Answer from the drawing. Dimensions are ordinates in mm from the lowest x, y and z of the part. A direction names the side the tool comes from. Coordinates: 2 decimals unless noted, no trailing zeros. Loops run counter-clockwise (first coordinate to the right, second up) from the corner with the lowest first, then second, coordinate; pieces in that order, holes last. Notation, with made-up numbers: (83, 68.25) -> (99, 68.25) arc R21 ccw to (99, 72.25) -> close; hole circle Ø2 at (-35, 59). An arc over 180 degrees is marked (long way). Use a Markdown table: item, result.
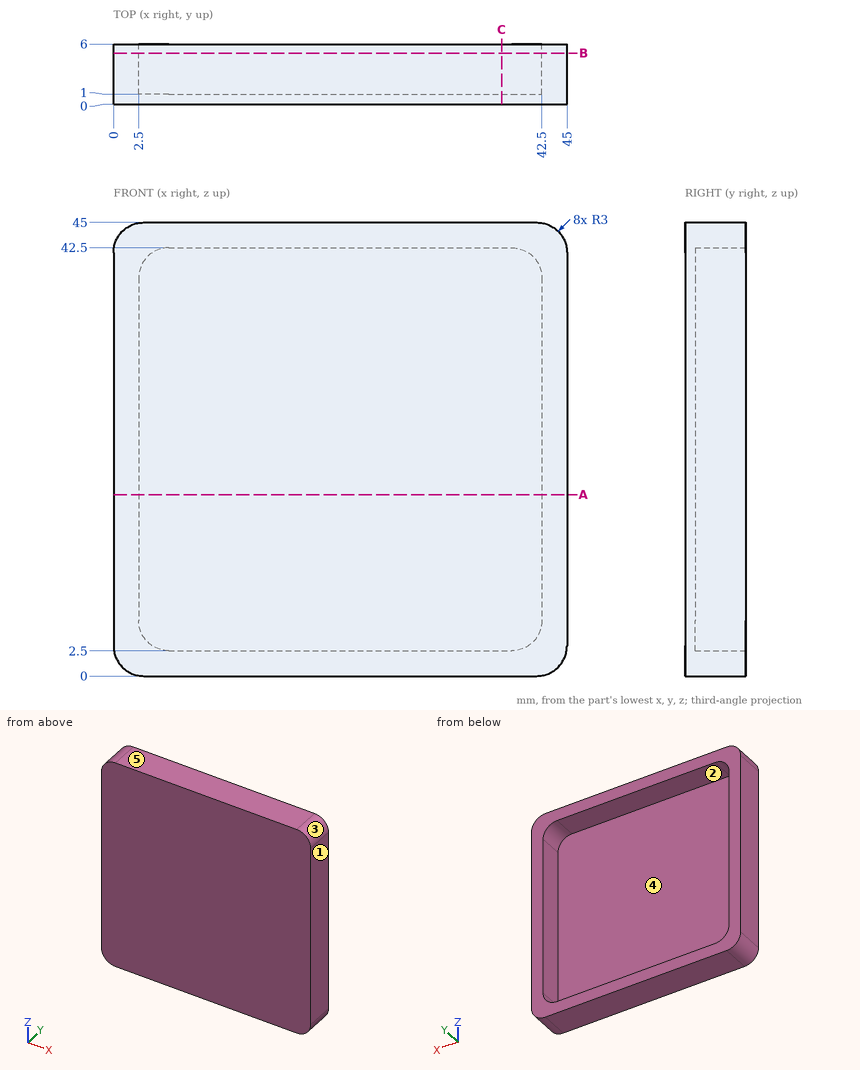
Q1. Section B-B on y = 5.1 is taken. Determine the outline of the cut face in (x, z), and give its area (3 significant figures).
Solved:
| item | result |
|---|---|
| outline | (0, 3) arc R3 ccw to (3, 0) -> (42, 0) arc R3 ccw to (45, 3) -> (45, 42) arc R3 ccw to (42, 45) -> (3, 45) arc R3 ccw to (0, 42) -> close; hole (2.5, 5.5) arc R3 ccw to (5.5, 2.5) -> (39.5, 2.5) arc R3 ccw to (42.5, 5.5) -> (42.5, 39.5) arc R3 ccw to (39.5, 42.5) -> (5.5, 42.5) arc R3 ccw to (2.5, 39.5) -> close |
| area | 425 mm² |
Q2. Section A-A on z = 18 is taken. Determine the outline of the cut face in (x, y).
Solved:
| item | result |
|---|---|
| outline | (0, 0) -> (45, 0) -> (45, 6) -> (42.5, 6) -> (42.5, 1) -> (2.5, 1) -> (2.5, 6) -> (0, 6) -> close |
Q3. Determine the mould class of the marked faces 1, 2 and 3 for opening direction Z: pulls with the +Z half, pulls with the -Z half, needs draft (parallel to the pull), parting line crosses it, or undercut.
Solved:
| item | result |
|---|---|
| face 1 | needs draft |
| face 2 | undercut |
| face 3 | pulls with the +Z half |
Q4. Consider line 1 (Z direction, x = 6, y = 1.8); line 2 (Y direction, x = 38, z = 42). Determine where each line is inside the solid, lowest interval first. Write a range as [from, to].
Solved:
| item | result |
|---|---|
| line 1 | [0, 2.5], [42.5, 45] |
| line 2 | [0, 1] |
Q5. For the marked faces 4 and 5, determine the directions among +Z, -Z, +X, -X, +Y, -Y from which every point of the face is accessible in a straight line to the end or side of a thin tool.
Solved:
| item | result |
|---|---|
| face 4 | +Y |
| face 5 | +Z, +X, -X, +Y, -Y |
Q6. Section C-C on x = 38.5 is taken. Determine the outline of the cut face in (y, z).
Solved:
| item | result |
|---|---|
| outline | (0, 0) -> (6, 0) -> (6, 2.5) -> (1, 2.5) -> (1, 42.5) -> (6, 42.5) -> (6, 45) -> (0, 45) -> close |
Q7. Given pin 1 Ø20 at (x, z) = (21.5, 22.5) entering from +Y, flat-ended and moving along its own axis, determine where the tip first touches the part or whether it passes through.
Solved:
| item | result |
|---|---|
| pin 1 | y = 1 |
